```python
from build123d import *

# Parameters (mm, degrees)
F0_W     = 46
F0_H     = 59
F1_DEPTH = 1
F0_W_2   = 47.6
F0_H_2   = 60.6
F2_DEPTH = 18
F3_W     = 4
F3_H     = 13.6829850562
F4_DEPTH = 100


with BuildPart() as f1:
    # F0 (on Top) → F1 (new body)
    with BuildSketch(Plane.XY):
        Rectangle(F0_W, F0_H)
    extrude(amount=F1_DEPTH)

    # F0 (on Top) → F2 (join)
    with BuildSketch(Plane.XY):
        Rectangle(F0_W_2, F0_H_2)
        Rectangle(F0_W, F0_H, mode=Mode.SUBTRACT)
    extrude(amount=F2_DEPTH)

    # F3 (on face) → F4 (cut)
    with BuildSketch(Plane.XZ.offset(30.3)):
        with Locations((-15, 11.1585074719)):
            Rectangle(F3_W, F3_H)
        with Locations((15, 11.1585074719)):
            Rectangle(F3_W, F3_H)
    extrude(amount=-F4_DEPTH, mode=Mode.SUBTRACT)


solid = f1.part
```
Build history of the part. All positions in model axes, mm. A direction names the side the tool comes from. Coordinates: 2 decimals unless noted, no trailing zeros. Order: outer loops, then holes, each group sorted by start corner. A loop starts at its lowest first (then second) coordinate and runs counter-clockwise, first axis right, second up. Notation, with made-up numbers: M -5.5,-35 L 39.5,-35 A24 ccw 39.5,-10 Z; hole C -21,-23.75 d2. An arc over 180 degrees is marked long. One line per question, with ' | ' between items. Start each with the question number.
1. Cut at C-C (x = -18.5). Write the cut outline in (y, z), plus the area to 3 significant figures.
2. Flat gauge pin, fed straight in: P1, Ø14, axis at x = -11.5, y = 10.5, coming from the +Z side. Where does the tip first touch, or does it go through?
3. Cut at B-B (y = -8.5). Write the cut outline in (x, z).
4. Wall check: line 1 along X through (y, z) = (6.5, 13); line 2 along Y through (x, z) = (11, 7.5); line 3 along Z through (x, y) = (18, 20). Give the ranges that are in metal, low to high. Write a range as [from, to].
5. Mould opens along X. For faces 3 (the face through (0, 29.5, 9)), 4 (the face through (23.4, 0.1, 18)), 5 (the face through (23.8, 0, 9)), 6 (the face through (-23, 0, 9)) say: +X half, -X half, draft (parallel to the pull), parting line (faces both ways), or undercut.
6. Tool access for faces 1 (the face through (0, -29.5, 9)), 2 (the face through (-23.8, 0, 9)): list every direction of +Z, -Z, +X, -X, +Y, -Y with a clear straight run to the whole face (end or side of a thin tool).
7. Cut at A-A (z = 7.25). Write the cut outline in (x, y), plus the area to 3 significant figures.
The answers:
1) outline: M -30.3,0 L 30.3,0 L 30.3,18 L 29.5,18 L 29.5,1 L -29.5,1 L -29.5,18 L -30.3,18 Z | area: 87.8 mm2
2) P1: stops at z = 1
3) outline: M -23.8,0 L 23.8,0 L 23.8,18 L 23,18 L 23,1 L -23,1 L -23,18 L -23.8,18 Z
4) line 1: x = [-23.8, -23], [23, 23.8] | line 2: y = [-30.3, -29.5], [29.5, 30.3] | line 3: z = [0, 1]
5) face 3: undercut | face 4: draft | face 5: +X half | face 6: undercut
6) face 1: +Z | face 2: +Z, -Z, -X, +Y, -Y
7) outline: M -23.8,-30.3 L -17,-30.3 L -17,-29.5 L -23,-29.5 L -23,29.5 L -17,29.5 L -17,30.3 L -23.8,30.3 Z; M -13,-30.3 L 13,-30.3 L 13,-29.5 L -13,-29.5 Z; M -13,29.5 L 13,29.5 L 13,30.3 L -13,30.3 Z; M 17,-30.3 L 23.8,-30.3 L 23.8,30.3 L 17,30.3 L 17,29.5 L 23,29.5 L 23,-29.5 L 17,-29.5 Z | area: 158 mm2
